from build123d import *

# Parameters (mm, degrees)
CHAMFER1_SIZE = 1
CHAMFER2_SIZE = 1


with BuildPart() as part:
    # Sketch1 → Revolve1 (revolve)
    with BuildSketch(Plane.ZY, mode=Mode.PRIVATE) as revolve1_sk:
        Polygon((-8, 3.5), (0, 3.5), (0, 15), (-3, 15), (-3, 5), (-8, 5), align=None)
    revolve(revolve1_sk.sketch.rotate(Axis((0, 0, 0), (0, 0, -1)), 90), axis=Axis((0, 0, 0), (0, 0, -1)))

    # Chamfer1
    chamfer1_edges = [part.edges().sort_by_distance(p)[0] for p in [
        (-5, 0, -8),
    ]]
    chamfer(chamfer1_edges, length=CHAMFER1_SIZE)

    # Chamfer2
    chamfer2_edges = [part.edges().sort_by_distance(p)[0] for p in [
        (-15, 0, 0),
        (-3.5, 0, 0),
    ]]
    chamfer(chamfer2_edges, length=CHAMFER2_SIZE)


solid = part.part
The model under review builds one solid part; all positions refer to its coordinate system, in mm. Coordinates: 2 decimals unless noted, no trailing zeros. Order: outer loops, then holes, each group sorted by start corner. A loop starts at its lowest first (then second) coordinate and runs counter-clockwise, first axis right, second up. Notation, with made-up numbers: (53, -24) -> (77, -24) arc R26 ccw to (77, 0) -> close; hole circle Ø6 at (-29.5, -29). An arc over 180 degrees is marked (long way). Answer in a Markdown table with one row per item.
(1) Consider section D-D (z = -6.5). Write out the cut boundary in (x, y), plus the area to 3 significant figures.
Answers:
| item | result |
|---|---|
| outline | circle Ø10 at (0, 0); hole circle Ø7 at (0, 0) |
| area | 40.1 mm² |
(2) Insertion check: pin 1 (4 mm diameter, centred on x = 7.5, y = -12, fed in from -Z); pin 2 (4 mm diameter, centred on x = 0, y = 0, fed in from +Z). Each pin has a flat end and moves straight along its axis. Give the tip position at first contact, or say it passes through.
Answers:
| item | result |
|---|---|
| pin 1 | z = -3 |
| pin 2 | through |
(3) Wall thickness on line 1 along Y through (x, z) = (0, -4.5); line 2 along Z through (x, y) = (-9.5, -4.25); line 3 along Y through (x, z) = (2, -4): over which ranges is each line inside the solid? List them lowest first.
Answers:
| item | result |
|---|---|
| line 1 | -5 to -3.5, 3.5 to 5 |
| line 2 | -3 to 0 |
| line 3 | -4.58 to -2.87, 2.87 to 4.58 |
(4) Consider section C-C (z = -1.75). Write out the cut boundary in (x, y), plus the area to 3 significant figures.
Answers:
| item | result |
|---|---|
| outline | circle Ø30 at (0, 0); hole circle Ø7 at (0, 0) |
| area | 668 mm² |
(5) The part is to be moulded in two halves that separate along Y. For faces 1 (the flat face through (3.3, -3.3, 0)), 2 (the cylindrical face through (1.615, 3.105, -4.451)), 3 (the cylindrical face through (8.06, -12.65, -2.01)), say which applies: +Y half, -Y half, draft (parallel to the pull), parting line (faces both ways), or undercut.
Answers:
| item | result |
|---|---|
| face 1 | draft |
| face 2 | undercut |
| face 3 | parting line |
(6) Consider section A-A (y = 0). Write out the cut boundary in (x, z).
Answers:
| item | result |
|---|---|
| outline | (-15, -3) -> (-5, -3) -> (-5, -7) -> (-4, -8) -> (-3.5, -8) -> (-3.5, -1) -> (-4.5, 0) -> (-14, 0) -> (-15, -1) -> close; (3.5, -8) -> (4, -8) -> (5, -7) -> (5, -3) -> (15, -3) -> (15, -1) -> (14, 0) -> (4.5, 0) -> (3.5, -1) -> close |
